Build history of the part. All positions in model axes, mm. A direction names the side the tool comes from. Round coordinates to 2 decimals unless told otherwise and drop trailing zeros. Loops run counter-clockwise (first coordinate to the right, second up) from the corner with the lowest first, then second, coordinate; pieces in that order, holes last.
from build123d import *

# Parameters (mm, degrees)
BOSS_EXTRUDE1_DEPTH = 12.7
FILLET1_R           = 2.54


with BuildPart() as part:
    # Sketch1 → Boss-Extrude1 (new body)
    with BuildSketch(Plane.XY):
        Polygon((0, 0), (0, 50.8), (25.4, 50.8), (25.4, 25.4), (44.45, 25.4), (44.45, 50.8), (63.5, 50.8), (63.5, 21.59), (88.9, 21.59), (88.9, 0), align=None)
    extrude(amount=BOSS_EXTRUDE1_DEPTH)

    # Fillet1
    fillet1_edges = [part.edges().sort_by_distance(p)[0] for p in [
        (0, 0, 6.35),
        (0, 50.8, 6.35),
        (25.4, 50.8, 6.35),
        (44.45, 50.8, 6.35),
        (63.5, 50.8, 6.35),
        (88.9, 21.59, 6.35),
        (88.9, 0, 6.35),
    ]]
    fillet(fillet1_edges, radius=FILLET1_R)


solid = part.part
(1) Pin check, flat tips, straight feed: P1, Ø6.5, axis at x = 35, z = 8.5, coming from the +Y side; P2, Ø4, axis at x = 77, z = 8.5, coming from the +Y side; P3, Ø6.5, axis at y = 33, z = 9, coming from the +X side. Stop position of each tip, or through.
Responses:
P1: stops at y = 25.4
P2: stops at y = 21.59
P3: stops at x = 63.5
(2) Slice it at D-D on x = 70. List the corners of the cut face in (y, z).
Responses:
outline: (0, 0) - (21.59, 0) - (21.59, 12.7) - (0, 12.7) - close
(3) Probe line 1 (X direction, y = 43.5, z = 9.25); line 2 (Y direction, x = 40, z = 1); line 3 (Y direction, x = 80, z = 10.5). List the from-to ranges inside material, lowest first.
Responses:
line 1: x = 0 to 25.4, 44.45 to 63.5
line 2: y = 0 to 25.4
line 3: y = 0 to 21.59
(4) Which spindle directions (+Z, -Z, +X, -X, +Y, -Y) get a long thin tool onto all of the face, cutting with end or side? Do faces 1 (the face through (25.4, 37, 6)), 2 (the face through (13, 50.8, 6)), 3 (the face through (75, 21.59, 6)). Say none if no direction does.
Responses:
face 1: +Z, -Z, +Y
face 2: +Z, -Z, +X, -X, +Y
face 3: +Z, -Z, +X, +Y
(5) Slice it at A-A on y = 31. List the corners of the cut face in (x, z), plus the area to 3 significant figures.
Responses:
outline: (0, 0) - (25.4, 0) - (25.4, 12.7) - (0, 12.7) - close; (44.45, 0) - (63.5, 0) - (63.5, 12.7) - (44.45, 12.7) - close
area: 565 mm2
(6) Slice it at C-C on x = 32. List the corners of the cut face in (y, z).
Responses:
outline: (0, 0) - (25.4, 0) - (25.4, 12.7) - (0, 12.7) - close
(7) Pull direction X, two halves, no side cores. Call faces 4 (the face through (62.736, 50.076, 6.439)), 5 (the face through (54, 50.8, 6)), 6 (the face through (44.45, 37, 6)): +X half, -X half, draft (parallel to the pull), parting line (faces both ways), or undercut.
Responses:
face 4: +X half
face 5: draft
face 6: undercut
(8) Slice it at B-B on z = 2. List the corners of the cut face in (x, y), plus the area to 3 significant figures.
Responses:
outline: (0, 2.54) arc R2.54 ccw to (2.54, 0) - (86.36, 0) arc R2.54 ccw to (88.9, 2.54) - (88.9, 19.05) arc R2.54 ccw to (86.36, 21.59) - (63.5, 21.59) - (63.5, 48.26) arc R2.54 ccw to (60.96, 50.8) - (46.99, 50.8) arc R2.54 ccw to (44.45, 48.26) - (44.45, 25.4) - (25.4, 25.4) - (25.4, 48.26) arc R2.54 ccw to (22.86, 50.8) - (2.54, 50.8) arc R2.54 ccw to (0, 48.26) - close
area: 3,280 mm2
